```python
from build123d import *

# Parameters (mm, degrees)
SKETCH001_R       = 0.65
PAD001_DEPTH      = 19.05
PAD001_DEPTH_BACK = 3.5
SKETCH_R          = 25.4
SKETCH_R_2        = 3.05
PAD_DEPTH         = 38.1
FILLET_R          = 0.5


with BuildPart() as pad001:
    # Sketch001 → Pad001 (new body, two sides)
    with BuildSketch(Plane.XY.offset(0.5)) as pad001_sk:
        Circle(SKETCH001_R)
        with Locations((33.27, 0)):
            Circle(SKETCH001_R)
    extrude(amount=PAD001_DEPTH)
    extrude(pad001_sk.sketch, amount=-PAD001_DEPTH_BACK)


with BuildPart() as obj1:
    # Sketch → Pad (new body)
    with BuildSketch(Plane.XY.offset(0.1)):
        with Locations((16.635, 0)):
            Circle(SKETCH_R)
        with Locations((16.635, 0)):
            Circle(SKETCH_R_2, mode=Mode.SUBTRACT)
    extrude(amount=PAD_DEPTH)

    # Fillet
    fillet_edges = [obj1.edges().sort_by_distance(p)[0] for p in [
        (13.585, 0, 38.2),
        (-8.765, 0, 38.2),
        (-8.765, 0, 0.1),
    ]]
    fillet(fillet_edges, radius=FILLET_R)

    # obj1: union Pad001
    add(pad001.part)


solid = obj1.part
```
Work out the finished part from the listing and answer in its coordinate system (mm). A direction names the side the tool comes from. Give positions to 0.01 mm unless a question says otherwise; leave off trailing zeros. Loops run counter-clockwise (first coordinate to the right, second up) from the corner with the lowest first, then second, coordinate; pieces in that order, holes last. Notation, with made-up numbers: (21.25, -3.75) - (27.25, -3.75) arc R24 ccw to (27.25, 28.25) - close; hole circle Ø4 at (-12.75, 40.5). An arc over 180 degrees is marked (long way). Use CSV: the item, a comma, the result in double quotes. Start each with the question number.
(1) Each of these flat-tipped pins is pushed along its axis until it touches: pin 1 (4 mm diameter, centred on x = -2, z = 6.5, fed in from -Y); pin 2 (5 mm diameter, centred on x = -1, z = 13.5, fed in from -Y); pin 3 (12 mm diameter, centred on x = 35.5, y = -19.5, fed in from -Z). Where does it stop, or does it pass through?
(2) Find the intervals of material crossed by L1, parallel to Y at x = 16.5, z = 25.5; L2, parallel to Z at x = 24, y = -22.5; L3, parallel to Y at x = 5.5, z = 6, in increasing order.
(3) Find section A-A, the plane z = 29. Determine the outline of the cut face in (x, y) (3 decimals), plus the area to 3 significant figures.
(4) A tool of negligible diameter and unlimited length cuts with its end or side. For faces 1 (the face through (-0.085, 0.644, -1.428)), 2 (the face through (0, 0, -3)), from which of +Z, -Z, +X, -X, +Y, -Y can it reach the whole face along a straight path? Write none if from no direction.
(5) Determine the mould class of faces 3 (the face through (-8.74, 1.12, 18.89)), 4 (the face through (13.588, 0.134, 18.637)), 5 (the face through (16, -5, 38.2)) for opening direction X: released by +X, released by -X, zero draft, split by the parting line, or undercut.
Results found:
1,pin 1,"y = -19.19"
1,pin 2,"y = -20.4"
1,pin 3,"z = 0.1"
2,L1,"-25.4 to -3.05, 3.05 to 25.4"
2,L2,"0.1 to 38.2"
2,L3,"-22.83 to 22.83"
3,outline,"circle Ø50.8 at (16.635, 0); hole circle Ø6.1 at (16.635, 0)"
3,area,"2,000 mm^2"
4,face 1,"-Z"
4,face 2,"-Z, +X, -X, +Y, -Y"
5,face 3,"split by the parting line"
5,face 4,"undercut"
5,face 5,"zero draft"
